Read the model definition and answer for the solid it produces. Units are mm, in the model's axes. A direction names the side the tool comes from. Coordinates: 2 decimals unless noted, no trailing zeros. Loops run counter-clockwise (first coordinate to the right, second up) from the corner with the lowest first, then second, coordinate; pieces in that order, holes last. Notation, with made-up numbers: (40.25, 74) - (86.25, 74) arc R25 ccw to (86.25, 99) - close; hole circle Ø10 at (-29, 55). An arc over 180 degrees is marked (long way). Use one line per item in the form item = value. Start each with the question number.
1) A cutting plane is placed at C-C (y = 21). Give the vertices of the cut face in (x, z).
2) Consider line 1 (Z direction, x = 4.25, y = 36); line 2 (Y direction, x = 7.25, z = -3). Determine where each line is inside the solid, lowest interval first.
3) Each of these flat-tipped pins is pushed along its axis until it touches: P1, Ø12.5, axis at x = 2, y = 31.5, coming from the -Z side; P2, Ø1.5, axis at x = -5.5, z = 15, coming from the +Y side; P3, Ø10, axis at x = -5, z = 5, coming from the -Y side. Where does it stop, or does it pass through?
4) A cutting plane is placed at D-D (x = 4). Give the vertices of the cut face in (y, z).
5) Which of the six approach directions +Z, -Z, +X, -X, +Y, -Y give full straight-line access (tool end or side, diameter ignored) to faces 1 (the face through (0, 8, 0)), 2 (the face through (12.7, 7.6, 10))?
6) A cutting plane is placed at A-A (x = 0). Give the vertices of the cut face in (y, z).
7) A cutting plane is placed at B-B (z = 0.5). Give the vertices of the cut face in (x, y), and give its area (3 significant figures).
from build123d import *

# Parameters (mm, degrees)
SKETCH1_W           = 25.4
SKETCH1_H           = 50
BOSS_EXTRUDE2_DEPTH = 8
BOSS_EXTRUDE4_DEPTH = 8


with BuildPart() as part:
    # Sketch1 → Boss-Extrude2 (new body)
    with BuildSketch(Plane(origin=(0, 0, 0), x_dir=(1, 0, 0), z_dir=(0, 1, 0))):
        Rectangle(SKETCH1_W, SKETCH1_H)
    extrude(amount=BOSS_EXTRUDE2_DEPTH)

    # Sketch4 → Boss-Extrude4 (add)
    with BuildSketch(Plane.XY.offset(25)):
        with BuildLine():
            Line((-12.7, 0), (12.7, 0))
            Line((12.7, 0), (12.7, 28))
            ThreePointArc((12.7, 28), (0, 40.7), (-12.7, 28))
            Line((-12.7, 28), (-12.7, 0))
        make_face()
    extrude(amount=BOSS_EXTRUDE4_DEPTH)


solid = part.part
Found:
q1.outline = (-12.7, 25) - (12.7, 25) - (12.7, 33) - (-12.7, 33) - close
q2.line_1 = 25 to 33
q2.line_2 = 0 to 8
q3.P1 = 25
q3.P2 = 8
q3.P3 = 0
q4.outline = (0, -25) - (8, -25) - (8, 25) - (40.05, 25) - (40.05, 33) - (0, 33) - close
q5.face_1 = -Z, +X, -X, +Y
q5.face_2 = +Z, -Z, +X, +Y, -Y
q6.outline = (0, -25) - (8, -25) - (8, 25) - (40.7, 25) - (40.7, 33) - (0, 33) - close
q7.outline = (-12.7, 0) - (12.7, 0) - (12.7, 8) - (-12.7, 8) - close
q7.area = 203 mm^2
